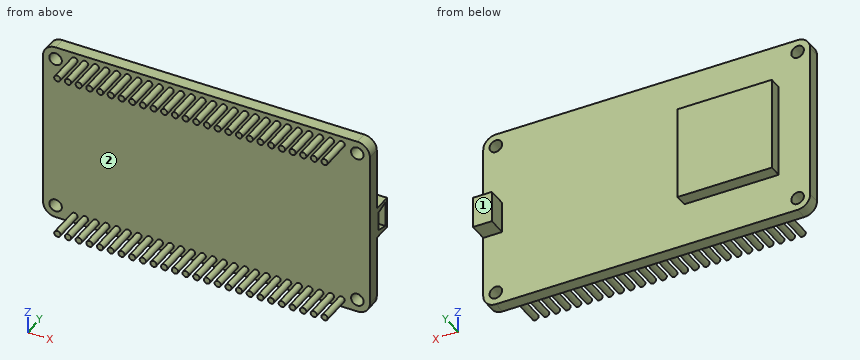
```python
from build123d import *

# Parameters (mm, degrees)
ESBO_O1_R                = 1
RESSALTO_EXTRUS_O1_DEPTH = 2
ESBO_O2_R                = 0.5
RESSALTO_EXTRUS_O2_DEPTH = 5
ESBO_O3_W                = 3
ESBO_O3_H                = 5
RESSALTO_EXTRUS_O3_DEPTH = 3
CORTE_EXTRUS_O1_DEPTH    = 2
ESBO_O5_W                = 15
ESBO_O5_H                = 15
RESSALTO_EXTRUS_O4_DEPTH = 2


with BuildPart() as part:
    # Esboço1 → Ressalto-extrusão1 (new body)
    with BuildSketch(Plane(origin=(0, 0, 0), x_dir=(1, 0, 0), z_dir=(0, 1, 0))):
        with BuildLine():
            Line((-25.276485788, 12.630490956), (22.723514212, 12.630490956))
            ThreePointArc((22.723514212, 12.630490956), (24.137727774, 12.044704518), (24.723514212, 10.630490956))
            Line((24.723514212, 10.630490956), (24.723514212, -14.369509044))
            ThreePointArc((24.723514212, -14.369509044), (24.137727774, -15.783722606), (22.723514212, -16.369509044))
            Line((22.723514212, -16.369509044), (-25.276485788, -16.369509044))
            ThreePointArc((-25.276485788, -16.369509044), (-26.69069935, -15.783722606), (-27.276485788, -14.369509044))
            Line((-27.276485788, -14.369509044), (-27.276485788, 10.630490956))
            ThreePointArc((-27.276485788, 10.630490956), (-26.69069935, 12.044704518), (-25.276485788, 12.630490956))
        make_face()
        with Locations((-25.276485788, 10.630490956)):
            Circle(ESBO_O1_R, mode=Mode.SUBTRACT)
        with Locations((-25.276485788, -14.369509044)):
            Circle(ESBO_O1_R, mode=Mode.SUBTRACT)
        with Locations((22.723514212, 10.630490956)):
            Circle(ESBO_O1_R, mode=Mode.SUBTRACT)
        with Locations((22.723514212, -14.369509044)):
            Circle(ESBO_O1_R, mode=Mode.SUBTRACT)
    extrude(amount=RESSALTO_EXTRUS_O1_DEPTH)

    # Esboço2 → Ressalto-extrusão2 (add)
    with BuildSketch(Plane.XZ):
        with Locations((-22.276485788, 15.14160434)):
            Circle(ESBO_O2_R)
        with Locations((-20.576485788, 15.14160434)):
            Circle(ESBO_O2_R)
        with Locations((-18.876485788, 15.14160434)):
            Circle(ESBO_O2_R)
        with Locations((-17.176485788, 15.14160434)):
            Circle(ESBO_O2_R)
        with Locations((-15.476485788, 15.14160434)):
            Circle(ESBO_O2_R)
        with Locations((-13.776485788, 15.14160434)):
            Circle(ESBO_O2_R)
        with Locations((-12.076485788, 15.14160434)):
            Circle(ESBO_O2_R)
        with Locations((-10.376485788, 15.14160434)):
            Circle(ESBO_O2_R)
        with Locations((-8.676485788, 15.14160434)):
            Circle(ESBO_O2_R)
        with Locations((-6.976485788, 15.14160434)):
            Circle(ESBO_O2_R)
        with Locations((-5.276485788, 15.14160434)):
            Circle(ESBO_O2_R)
        with Locations((-3.576485788, 15.14160434)):
            Circle(ESBO_O2_R)
        with Locations((-1.876485788, 15.14160434)):
            Circle(ESBO_O2_R)
        with Locations((-0.176485788, 15.14160434)):
            Circle(ESBO_O2_R)
        with Locations((1.523514212, 15.14160434)):
            Circle(ESBO_O2_R)
        with Locations((3.223514212, 15.14160434)):
            Circle(ESBO_O2_R)
        with Locations((4.923514212, 15.14160434)):
            Circle(ESBO_O2_R)
        with Locations((6.623514212, 15.14160434)):
            Circle(ESBO_O2_R)
        with Locations((8.323514212, 15.14160434)):
            Circle(ESBO_O2_R)
        with Locations((10.023514212, 15.14160434)):
            Circle(ESBO_O2_R)
        with Locations((11.723514212, 15.14160434)):
            Circle(ESBO_O2_R)
        with Locations((13.423514212, 15.14160434)):
            Circle(ESBO_O2_R)
        with Locations((15.123514212, 15.14160434)):
            Circle(ESBO_O2_R)
        with Locations((16.823514212, 15.14160434)):
            Circle(ESBO_O2_R)
        with Locations((18.523514212, 15.14160434)):
            Circle(ESBO_O2_R)
        with Locations((20.223514212, 15.14160434)):
            Circle(ESBO_O2_R)
        with Locations((-22.276485788, -11.402586252)):
            Circle(ESBO_O2_R)
        with Locations((-20.576485788, -11.402586252)):
            Circle(ESBO_O2_R)
        with Locations((-18.876485788, -11.402586252)):
            Circle(ESBO_O2_R)
        with Locations((-17.176485788, -11.402586252)):
            Circle(ESBO_O2_R)
        with Locations((-15.476485788, -11.402586252)):
            Circle(ESBO_O2_R)
        with Locations((-13.776485788, -11.402586252)):
            Circle(ESBO_O2_R)
        with Locations((-12.076485788, -11.402586252)):
            Circle(ESBO_O2_R)
        with Locations((-10.376485788, -11.402586252)):
            Circle(ESBO_O2_R)
        with Locations((-8.676485788, -11.402586252)):
            Circle(ESBO_O2_R)
        with Locations((-6.976485788, -11.402586252)):
            Circle(ESBO_O2_R)
        with Locations((-5.276485788, -11.402586252)):
            Circle(ESBO_O2_R)
        with Locations((-3.576485788, -11.402586252)):
            Circle(ESBO_O2_R)
        with Locations((-1.876485788, -11.402586252)):
            Circle(ESBO_O2_R)
        with Locations((-0.176485788, -11.402586252)):
            Circle(ESBO_O2_R)
        with Locations((1.523514212, -11.402586252)):
            Circle(ESBO_O2_R)
        with Locations((3.223514212, -11.402586252)):
            Circle(ESBO_O2_R)
        with Locations((4.923514212, -11.402586252)):
            Circle(ESBO_O2_R)
        with Locations((6.623514212, -11.402586252)):
            Circle(ESBO_O2_R)
        with Locations((8.323514212, -11.402586252)):
            Circle(ESBO_O2_R)
        with Locations((10.023514212, -11.402586252)):
            Circle(ESBO_O2_R)
        with Locations((11.723514212, -11.402586252)):
            Circle(ESBO_O2_R)
        with Locations((13.423514212, -11.402586252)):
            Circle(ESBO_O2_R)
        with Locations((15.123514212, -11.402586252)):
            Circle(ESBO_O2_R)
        with Locations((16.823514212, -11.402586252)):
            Circle(ESBO_O2_R)
        with Locations((18.523514212, -11.402586252)):
            Circle(ESBO_O2_R)
        with Locations((20.223514212, -11.402586252)):
            Circle(ESBO_O2_R)
    extrude(amount=RESSALTO_EXTRUS_O2_DEPTH)

    # Esboço3 → Ressalto-extrusão3 (add)
    with BuildSketch(Plane(origin=(0, 2, 0), x_dir=(1, 0, 0), z_dir=(0, 1, 0))):
        with Locations((23.223514212, -1.869509044)):
            Rectangle(ESBO_O3_W, ESBO_O3_H)
    extrude(amount=RESSALTO_EXTRUS_O3_DEPTH)

    # Esboço4 → Corte-extrusão1 (cut)
    with BuildSketch(Plane(origin=(24.723514212, 0, 0), x_dir=(0, 0, -1), z_dir=(1, 0, 0))):
        Polygon((0.130490956, 4.5), (-0.369509044, 2.5), (-3.369509044, 2.5), (-3.869509044, 4.5), align=None)
    extrude(amount=-CORTE_EXTRUS_O1_DEPTH, mode=Mode.SUBTRACT)

    # Esboço5 → Ressalto-extrusão4 (add)
    with BuildSketch(Plane(origin=(0, 2, 0), x_dir=(1, 0, 0), z_dir=(0, 1, 0))):
        with Locations((-14.764317849, -1.869509044)):
            Rectangle(ESBO_O5_W, ESBO_O5_H)
    extrude(amount=RESSALTO_EXTRUS_O4_DEPTH)


solid = part.part
```
The model under review builds one solid part; all positions refer to its coordinate system, in mm. Face numbers are marked on the shaded views. Coordinates: 2 decimals unless noted, no trailing zeros. Loops run counter-clockwise (first coordinate to the right, second up) from the corner with the lowest first, then second, coordinate; pieces in that order, holes last. Notation, with made-up numbers: (-16.5, -8) -> (32.5, -8) arc R23 cw to (32.5, 17) -> close; hole circle Ø3 at (18, -27). An arc over 180 degrees is marked (long way). Answer as CSV lines item,"result".
Item 1: Insertion check: pin 1 (8 mm diameter, centred on x = 17.5, z = 4, fed in from +Y); pin 2 (5 mm diameter, centred on y = -3.5, z = -9.5, fed in from -X); pin 3 (2.5 mm diameter, centred on x = 22.72, z = 14.37, fed in from -Y). Each pin has a flat end and moves straight along its axis. Give the tip position at first contact, or say it passes through.
Results below:
pin 1,"stops at y = 2"
pin 2,"stops at x = -22.78"
pin 3,"stops at y = 0"
Item 2: Draft analysis for pull direction Z (two halves, no side actions). For the marked faces 1 and 2, state which applies: +Z half, -Z half, draft (parallel to the pull), parting line (faces both ways), or undercut.
Results below:
face 1,"draft"
face 2,"undercut"
Item 3: Take a section at A-A, the plane y = 3. State the section outline as (x, z) points.
Results below:
outline,"(-22.26, -5.63) -> (-7.26, -5.63) -> (-7.26, 9.37) -> (-22.26, 9.37) -> close; (21.72, -0.63) -> (24.72, -0.63) -> (24.72, 0.24) -> (22.72, 0.24) -> (22.72, 3.49) -> (24.72, 3.49) -> (24.72, 4.37) -> (21.72, 4.37) -> close"
Item 4: Take a section at C-C, the plane y = -2. Count the separate pieces of the cut face and the enclosed holes in it, and give its area (3 significant figures).
Results below:
separate pieces,"52"
enclosed holes,"0"
area,"40.8 mm2"
Item 5: For L1, parallel to Y at x = -11.5, z = 14.5; L2, parallel to Y at x = -22, z = -1.25; L3, parallel to Z at x = -19, y = -3.75, list the stretches that pass through material, from the lowest coordinate up.
Results below:
L1,"y = 0 to 2"
L2,"y = 0 to 4"
L3,"z = -11.89 to -10.92, 14.66 to 15.63"
Item 6: Take a section at B-B, the plane z = 5.75. State the section outline as (x, y) points.
Results below:
outline,"(-27.28, 0) -> (24.72, 0) -> (24.72, 2) -> (-7.26, 2) -> (-7.26, 4) -> (-22.26, 4) -> (-22.26, 2) -> (-27.28, 2) -> close"
